from build123d import *

# Parameters (mm, degrees)
SKETCH1_R           = 8.7
SKETCH1_R_2         = 5.5
BOSS_EXTRUDE1_DEPTH = 68.8
BOSS_EXTRUDE2_START = 4
SKETCH2_R           = 16
SKETCH2_R_2         = 5.5
BOSS_EXTRUDE2_DEPTH = 4
FILLET1_R           = 2
FILLET2_R           = 1
BOSS_EXTRUDE6_START = -10
BOSS_EXTRUDE6_DEPTH = 10
CUT_EXTRUDE1_START  = -23
SKETCH10_R          = 8.7
SKETCH10_R_2        = 7.2
CUT_EXTRUDE1_DEPTH  = 23
SKETCH11_R          = 18.546055896
CUT_EXTRUDE2_DEPTH  = 54.972215104
SKETCH12_R          = 7.3
CUT_EXTRUDE3_DEPTH  = 15


with BuildPart() as part:
    # Sketch1 → Boss-Extrude1 (new body)
    with BuildSketch(Plane(origin=(0, 0, 0), x_dir=(1, 0, 0), z_dir=(0, 1, 0))):
        with Locations(Location((0, 0, 0), (0, 0, 90))):
            Circle(SKETCH1_R)
        with Locations(Location((0, 0, 0), (0, 0, 90))):
            Circle(SKETCH1_R_2, mode=Mode.SUBTRACT)
    extrude(amount=BOSS_EXTRUDE1_DEPTH)

    # Sketch2 → Boss-Extrude2 (add)
    with BuildSketch(Plane.XZ.offset(BOSS_EXTRUDE2_START)):
        with Locations(Location((0, 0, 0), (0, 0, 270))):
            Circle(SKETCH2_R)
        with Locations(Location((0, 0, 0), (0, 0, 270))):
            Circle(SKETCH2_R_2, mode=Mode.SUBTRACT)
    extrude(amount=-BOSS_EXTRUDE2_DEPTH)

    # Fillet1
    fillet1_edges = [part.edges().sort_by_distance(p)[0] for p in [
        (0, 0, 16),
        (0, -4, 16),
    ]]
    fillet(fillet1_edges, radius=FILLET1_R - 0.0001)  # a hair under: the kernel refuses the full size

    # Fillet2
    fillet2_edges = [part.edges().sort_by_distance(p)[0] for p in [
        (0, 0, 8.7),
    ]]
    fillet(fillet2_edges, radius=FILLET2_R)

    # Sketch7 → Boss-Extrude6 (add)
    with BuildSketch(Plane(origin=(0, 68.8, 0), x_dir=(1, 0, 0), z_dir=(0, 1, 0)).offset(BOSS_EXTRUDE6_START)):
        with BuildLine():
            Line((-8.459778344, -2.030307951), (-9.805994948, -2.807572454))
            ThreePointArc((-9.805994948, -2.807572454), (-8.832386986, -5.101856537), (-7.331446138, -7.091537035))
            Line((-7.331446138, -7.091537035), (-5.988187435, -6.311228981))
            ThreePointArc((-5.988187435, -6.311228981), (-7.534421013, -4.35), (-8.459778344, -2.030307951))
        make_face()
        with BuildLine():
            Line((-2.471590909, 8.341536931), (-2.475728155, 9.89498712))
            ThreePointArc((-2.475728155, 9.89498712), (0, 10.2), (2.475728155, 9.89498712))
            Line((2.475728155, 9.89498712), (2.471590909, 8.341536931))
            ThreePointArc((2.471590909, 8.341536931), (0, 8.7), (-2.471590909, 8.341536931))
        make_face()
        with BuildLine():
            Line((8.459778344, -2.030307951), (9.807174294, -2.803450085))
            ThreePointArc((9.807174294, -2.803450085), (8.833459119, -5.1), (7.331446138, -7.091537035))
            Line((7.331446138, -7.091537035), (5.988187435, -6.311228981))
            ThreePointArc((5.988187435, -6.311228981), (7.534421013, -4.35), (8.459778344, -2.030307951))
        make_face()
    extrude(amount=BOSS_EXTRUDE6_DEPTH)

    # Sketch10 → Cut-Extrude1 (cut)
    with BuildSketch(Plane(origin=(0, 45, 0), x_dir=(1, 0, 0), z_dir=(0, 1, 0)).offset(CUT_EXTRUDE1_START)):
        with Locations(Location((0, 0, 0), (0, 0, 90))):
            Circle(SKETCH10_R)
        with Locations(Location((0, 0, 0), (0, 0, 270))):
            Circle(SKETCH10_R_2, mode=Mode.SUBTRACT)
    extrude(amount=CUT_EXTRUDE1_DEPTH, mode=Mode.SUBTRACT)

    # Sketch11 → Cut-Extrude2 (cut, through all)
    with BuildSketch(Plane.XZ.offset(-45)):
        Circle(SKETCH11_R)
    extrude(amount=CUT_EXTRUDE2_DEPTH, mode=Mode.SUBTRACT)

    # Sketch12 → Cut-Extrude3 (cut)
    with BuildSketch(Plane.XZ.offset(-45)):
        with Locations(Location((0, 0, 0), (0, 0, 270))):
            Circle(SKETCH12_R)
    extrude(amount=-CUT_EXTRUDE3_DEPTH, mode=Mode.SUBTRACT)


solid = part.part
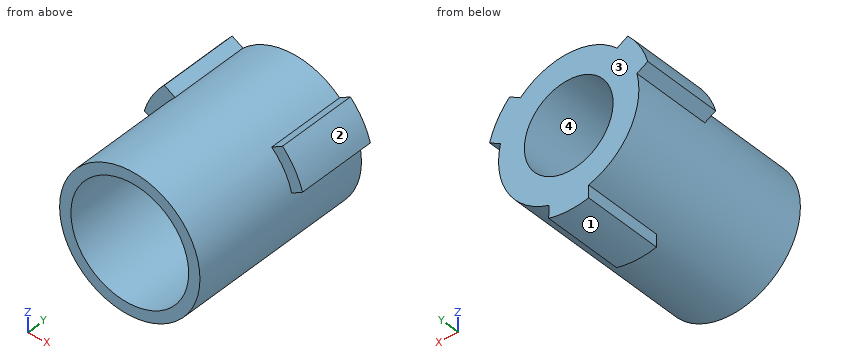
Design review of the part built by this model. Coordinates are the model's own, in mm. Face numbers are marked on the shaded views. Coordinates: 2 decimals unless noted, no trailing zeros. Order: outer loops, then holes, each group sorted by start corner. A loop starts at its lowest first (then second) coordinate and runs counter-clockwise, first axis right, second up. Notation, with made-up numbers: (-38.75, -2.75) -> (-32.75, -2.75) arc R25 cw to (-32.75, 30.25) -> close; hole circle Ø8 at (13.5, 86.25). An arc over 180 degrees is marked (long way). Use one line per item in the form item = value. Start each with the question number.
(1) Add section D-D on x = 3.25. State the section outline as (y, z) points, plus the area to 3 significant figures.
(2) The part is to be moulded in two halves that separate along X. For the marked faces 1, 2, 3 and 4, say which applies: +X half, -X half, draft (parallel to the pull), parting line (faces both ways), or undercut.
(3) Add section C-C on y = 61. State the section outline as (x, z) points.
(4) Add section A-A on x = 0. State the section outline as (y, z) points.
(5) Insertion check: pin 1 (1.9 mm diameter, centred on x = -8, z = 4.5, fed in from -Y); pin 2 (6 mm diameter, centred on x = 6.5, y = 51.5, fed in from -Z); pin 3 (4 mm diameter, centred on y = 49.5, z = 4, fed in from -X); pin 4 (6 mm diameter, centred on y = 66, z = -7.5, fed in from +X). Each pin has a flat end and moves straight along its axis. Give the tip position at first contact, or say it passes through.
(6) Add section B-B on z = 0. State the section outline as (x, y) points, plus the area to 3 significant figures.
(7) For probe 1 along X at (y, z) = (50, 0); probe 2 along X at (y, z) = (63.75, 0); probe 3 along Z at (x, y) = (-3, 68.25), list the stretches that pass through material, from the lowest coordinate up.
Answer block:
q1.outline = (45, -8.07) -> (68.8, -8.07) -> (68.8, -4.44) -> (60, -4.44) -> (60, -6.54) -> (45, -6.54) -> close; (45, 6.54) -> (60, 6.54) -> (60, 4.44) -> (68.8, 4.44) -> (68.8, 8.07) -> (45, 8.07) -> close
q1.area = 110 mm²
q2.face_1 = parting line
q2.face_2 = +X half
q2.face_3 = draft
q2.face_4 = undercut
q3.outline = (-9.81, 2.81) -> (-8.46, 2.03) arc R8.7 ccw to (-2.47, -8.34) -> (-2.48, -9.89) arc R10.2 ccw to (2.48, -9.89) -> (2.47, -8.34) arc R8.7 ccw to (8.46, 2.03) -> (9.81, 2.8) arc R10.2 ccw to (7.33, 7.09) -> (5.99, 6.31) arc R8.7 ccw to (-5.99, 6.31) -> (-7.33, 7.09) arc R10.2 ccw to start; hole circle Ø11 at (0, 0)
q4.outline = (45, -8.7) -> (58.8, -8.7) -> (58.8, -10.2) -> (68.8, -10.2) -> (68.8, -5.5) -> (60, -5.5) -> (60, -7.3) -> (45, -7.3) -> close; (45, 7.3) -> (60, 7.3) -> (60, 5.5) -> (68.8, 5.5) -> (68.8, 8.7) -> (45, 8.7) -> close
q5.pin_1 = 45
q5.pin_2 = -7.96
q5.pin_3 = -8.47
q5.pin_4 = 7.45
q6.outline = (-8.7, 45) -> (-7.3, 45) -> (-7.3, 60) -> (-5.5, 60) -> (-5.5, 68.8) -> (-8.7, 68.8) -> close; (5.5, 60) -> (7.3, 60) -> (7.3, 45) -> (8.7, 45) -> (8.7, 68.8) -> (5.5, 68.8) -> close
q6.area = 98.3 mm²
q7.probe_1 = -8.7 to -7.3, 7.3 to 8.7
q7.probe_2 = -8.7 to -5.5, 5.5 to 8.7
q7.probe_3 = -8.17 to -4.61, 4.61 to 8.17
